Check sheet for the drawn part. Datum: minimum x, y, z corner. Units: mm. Coordinates: 2 decimals unless noted, no trailing zeros. Loops run counter-clockwise (first coordinate to the right, second up) from the corner with the lowest first, then second, coordinate; pieces in that order, holes last.
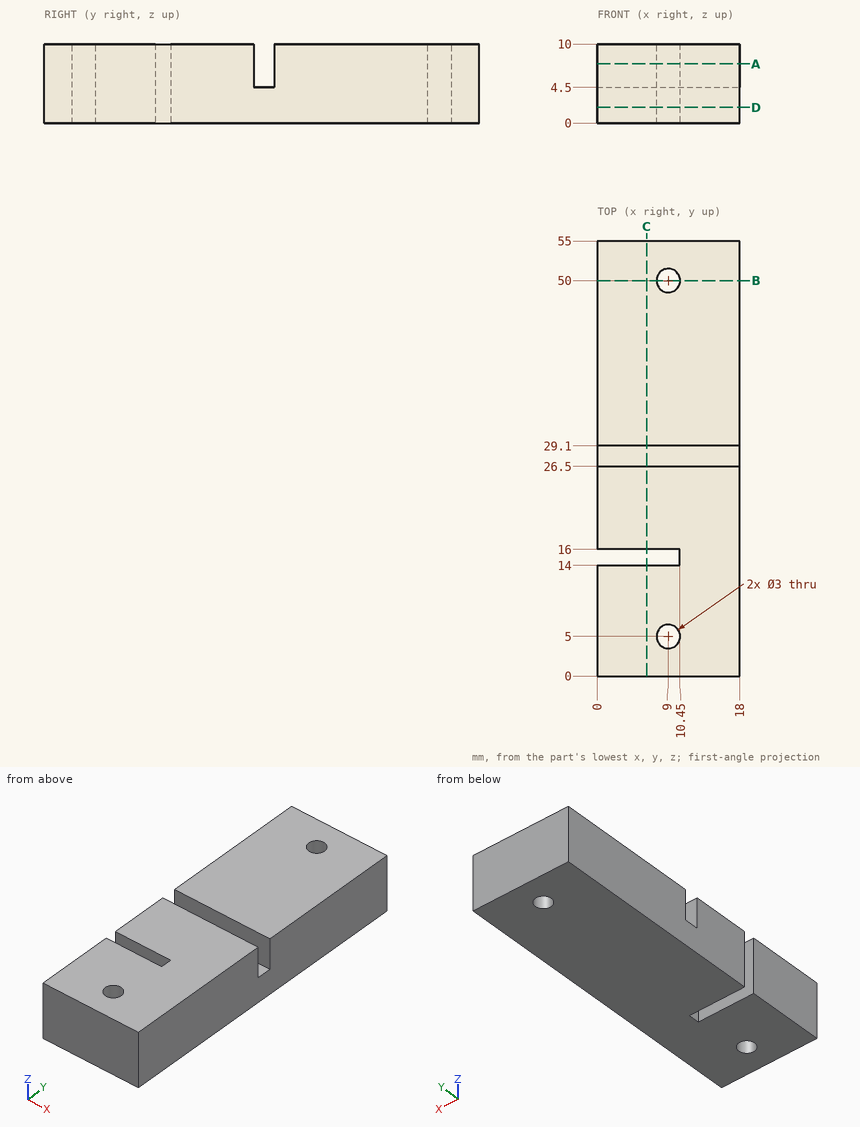
1) Section check C-C on x = 6.25. Enter the section's corners in (y, z).
Answer sheet:
outline: (0, 0) - (14, 0) - (14, 10) - (0, 10) - close; (16, 0) - (55, 0) - (55, 10) - (29.1, 10) - (29.1, 4.5) - (26.5, 4.5) - (26.5, 10) - (16, 10) - close
2) Depth check by flat-ended pin: pin 1 (4 mm diameter, centred on x = 9, y = 50, fed in from +Z); pin 2 (1.6 mm diameter, centred on y = 15, z = 5.5, fed in from -X); pin 3 (2 mm diameter, centred on x = 5, y = 28, fed in from +Z); pin 4 (1.8 mm diameter, centred on x = 9, y = 5, fed in from +Z). Enter the tip coordinate at first touch or a pass-through.
Answer sheet:
pin 1: stops at z = 10
pin 2: stops at x = 10.45
pin 3: stops at z = 4.5
pin 4: passes through
3) Section check B-B on y = 50. Enter the section's corners in (x, z), plus the area to 3 significant figures.
Answer sheet:
outline: (0, 0) - (7.5, 0) - (7.5, 10) - (0, 10) - close; (10.5, 0) - (18, 0) - (18, 10) - (10.5, 10) - close
area: 150 mm2
4) Section check D-D on z = 2. Enter the section's corners in (x, y), plus the area to 3 significant figures.
Answer sheet:
outline: (0, 0) - (18, 0) - (18, 55) - (0, 55) - (0, 16) - (10.45, 16) - (10.45, 14) - (0, 14) - close; hole circle Ø3 at (9, 5); hole circle Ø3 at (9, 50)
area: 955 mm2
5) Scan lines: line 1 (Y direction, x = 9, z = 3.75); line 2 (Y direction, x = 6.5, z = 5.5); line 3 (Y direction, x = 9, z = 5). Record each from-to range of solid material in increasing order.
Answer sheet:
line 1: y = 0 to 3.5, 6.5 to 14, 16 to 48.5, 51.5 to 55
line 2: y = 0 to 14, 16 to 26.5, 29.1 to 55
line 3: y = 0 to 3.5, 6.5 to 14, 16 to 26.5, 29.1 to 48.5, 51.5 to 55
6) Section check A-A on z = 7.5. Enter the section's corners in (x, y), plus the area to 3 significant figures.
Answer sheet:
outline: (0, 0) - (18, 0) - (18, 26.5) - (0, 26.5) - (0, 16) - (10.45, 16) - (10.45, 14) - (0, 14) - close; (0, 29.1) - (18, 29.1) - (18, 55) - (0, 55) - close; hole circle Ø3 at (9, 5); hole circle Ø3 at (9, 50)
area: 908 mm2
